from build123d import *

# Parameters (mm, degrees)
ESBO_O1_W                = 28.5
ESBO_O1_H                = 12
ESBO_O1_R                = 3
RESSALTO_EXTRUS_O1_DEPTH = 36
ESBO_O2_W                = 10
ESBO_O2_H                = 45
CORTE_EXTRUS_O1_DEPTH    = 10
FILETE1_R                = 0.5


with BuildPart() as part:
    # Esboço1 → Ressalto-extrusão1 (new, symmetric)
    with BuildSketch(Plane(origin=(0, 0, 0), x_dir=(1, 0, 0), z_dir=(0, 1, 0))):
        Rectangle(ESBO_O1_W, ESBO_O1_H)
        with Locations(Location((6.205688, 0, 0), (0, 0, 270))):
            Circle(ESBO_O1_R, mode=Mode.SUBTRACT)
    extrude(amount=RESSALTO_EXTRUS_O1_DEPTH, both=True)

    # Esboço2 → Corte-extrusão1 (cut, symmetric)
    with BuildSketch(Plane.XY):
        with Locations((-14.25, 0)):
            Rectangle(ESBO_O2_W, ESBO_O2_H)
        with Locations((14.25, 0)):
            Rectangle(ESBO_O2_W, ESBO_O2_H)
    extrude(amount=CORTE_EXTRUS_O1_DEPTH, both=True, mode=Mode.SUBTRACT)

    # Filete1
    filete1_edges = [part.edges().sort_by_distance(p)[0] for p in [
        (-14.25, 36, 0),
        (6.205688, -36, -3),
        (6.205688, 36, -3),
        (0, 36, 6),
        (-14.25, -29.25, 6),
        (-11.75, 22.5, 6),
        (-9.25, 0, 6),
        (-11.75, -22.5, 6),
        (-14.25, -29.25, -6),
        (-9.25, 0, -6),
        (-14.25, -22.5, 0),
        (-11.75, -22.5, -6),
        (-11.75, 22.5, -6),
        (-14.25, 22.5, 0),
        (14.25, -29.25, 6),
        (11.75, 22.5, 6),
        (9.25, 0, 6),
        (11.75, -22.5, 6),
        (14.25, -29.25, -6),
        (11.75, -22.5, -6),
        (14.25, 36, 0),
        (14.25, -22.5, 0),
        (9.25, 0, -6),
        (14.25, 22.5, 0),
        (11.75, 22.5, -6),
        (0, -36, 6),
        (-14.25, -36, 0),
        (0, -36, -6),
        (14.25, -36, 0),
        (0, 36, -6),
        (14.25, 29.25, 6),
        (-14.25, 29.25, 6),
        (-14.25, 29.25, -6),
        (14.25, 29.25, -6),
    ]]
    fillet(filete1_edges, radius=FILETE1_R)


solid = part.part
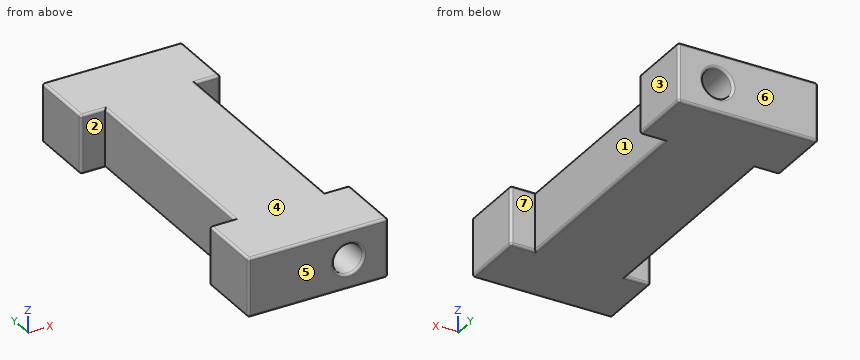
CAD build for the part. Positions are in the model's coordinates, mm. Face numbers are marked on the shaded views. A direction names the side the tool comes from. Round coordinates to 2 decimals unless told otherwise and drop trailing zeros. Write each loop counter-clockwise with the first axis right and the second up, starting at its lowest first coordinate (ties: lowest second). Pieces come first, ordered by that corner, then holes. Notation, with made-up numbers: (56.25, 70) -> (75.25, 70) arc R31 ccw to (75.25, 109) -> close; hole circle Ø7 at (80.5, 23). An arc over 180 degrees is marked (long way). Answer as a JSON object with one key per item and string values.
(1) Band-saw the part on B-B, the plane x = 11.25. List the corners of the cut face in (y, z).
Reported:
{"outline": "(-36, -5.5) arc R0.5 ccw to (-35.5, -6) -> (-23, -6) arc R0.5 ccw to (-22.5, -5.5) -> (-22.5, 5.5) arc R0.5 ccw to (-23, 6) -> (-35.5, 6) arc R0.5 ccw to (-36, 5.5) -> close; (22.5, -5.5) arc R0.5 ccw to (23, -6) -> (35.5, -6) arc R0.5 ccw to (36, -5.5) -> (36, 5.5) arc R0.5 ccw to (35.5, 6) -> (23, 6) arc R0.5 ccw to (22.5, 5.5) -> close"}
(2) Which spindle directions (+Z, -Z, +X, -X, +Y, -Y) get a long thin tool onto all of the face, cutting with end or side? Do the marked faces 1, 2 and 3. Say none if no direction does.
Reported:
{"face 1": "+Z, -Z, +X", "face 2": "+Z, -Z, -X", "face 3": "+Z, -Z, +X, +Y, -Y"}
(3) Band-saw the part on D-D, the plane y = -17.5. List the corners of the cut face in (x, z).
Reported:
{"outline": "(-9.25, -5.5) arc R0.5 ccw to (-8.75, -6) -> (8.75, -6) arc R0.5 ccw to (9.25, -5.5) -> (9.25, 5.5) arc R0.5 ccw to (8.75, 6) -> (-8.75, 6) arc R0.5 ccw to (-9.25, 5.5) -> close; hole circle Ø6 at (6.21, 0)"}
(4) Band-saw the part on A-A, the plane z = 0. List the corners of the cut face in (x, y), then the cut area to 3 significant figures.
Reported:
{"outline": "(-14.25, -35.5) arc R0.5 ccw to (-13.75, -36) -> (2.71, -36) arc R0.5 ccw to (3.21, -35.5) -> (3.21, 35.5) arc R0.5 ccw to (2.71, 36) -> (-13.75, 36) arc R0.5 ccw to (-14.25, 35.5) -> (-14.25, 23) arc R0.5 ccw to (-13.75, 22.5) -> (-9.25, 22.5) -> (-9.25, -22.5) -> (-13.75, -22.5) arc R0.5 ccw to (-14.25, -23) -> close; (9.21, -35.5) arc R0.5 ccw to (9.71, -36) -> (13.75, -36) arc R0.5 ccw to (14.25, -35.5) -> (14.25, -23) arc R0.5 ccw to (13.75, -22.5) -> (9.25, -22.5) -> (9.25, 22.5) -> (13.75, 22.5) arc R0.5 ccw to (14.25, 23) -> (14.25, 35.5) arc R0.5 ccw to (13.75, 36) -> (9.71, 36) arc R0.5 ccw to (9.21, 35.5) -> close", "area": "1,170 mm^2"}
(5) Band-saw the part on C-C, the plane y = -29. List the corners of the cut face in (x, z), then the cut area to 3 significant figures.
Reported:
{"outline": "(-14.25, -5.5) arc R0.5 ccw to (-13.75, -6) -> (13.75, -6) arc R0.5 ccw to (14.25, -5.5) -> (14.25, 5.5) arc R0.5 ccw to (13.75, 6) -> (-13.75, 6) arc R0.5 ccw to (-14.25, 5.5) -> close; hole circle Ø6 at (6.21, 0)", "area": "314 mm^2"}
(6) Pin check, flat tips, straight feed: P1, Ø1.5, axis at y = -6.5, z = -3.5, coming from the +X side; P2, Ø1, axis at x = 7, z = 0, coming from the +Y side; P3, Ø4, axis at y = 10.5, z = 3, coming from the -X side. Stop position of each tip, or through.
Reported:
{"P1": "stops at x = 9.25", "P2": "passes through", "P3": "stops at x = -9.25"}
(7) Probe probe 1 along Y at (x, z) = (-10.75, -3); probe 2 along Z at (x, y) = (7.5, -15); probe 3 along X at (y, z) = (-20.5, 3.5). List the from-to ranges inside material, lowest first. Write a range as [from, to].
Reported:
{"probe 1": "y = [-36, -22.5], [22.5, 36]", "probe 2": "z = [-6, -2.71], [2.71, 6]", "probe 3": "x = [-9.25, 9.25]"}
(8) Two-plate mould, pull along Y, no slides. Class the marked faces 4, 5, 6 and 7: +Y half, -Y half, draft (parallel to the pull), parting line (faces both ways), or undercut.
Reported:
{"face 4": "draft", "face 5": "-Y half", "face 6": "+Y half", "face 7": "undercut"}
